from build123d import *


with BuildPart() as part:
    # Esquisse1 → Révolution1 (revolve)
    with BuildSketch(Plane.XY, mode=Mode.PRIVATE) as r_volution1_sk:
        Polygon((0, 45.2), (0, 50.8), (-0.2, 51), (-22.267949192, 51), (-24, 54), (-24, 67.8), (-24.2, 68), (-37.8, 68), (-38, 67.8), (-38, 58), (-47.8, 58), (-48, 57.8), (-48, 45.2), (-47.8, 45), (-0.2, 45), align=None)
    revolve(r_volution1_sk.sketch.rotate(Axis((0, 0, 0), (-1, 0, 0)), 90), axis=Axis((0, 0, 0), (-1, 0, 0)))  # turned: the seam where the file's is


solid = part.part
Model file for the job. Use its own axes, mm. A direction names the side the tool comes from. Give positions to 0.01 mm unless a question says otherwise; leave off trailing zeros. Write each loop counter-clockwise with the first axis right and the second up, starting at its lowest first coordinate (ties: lowest second). Pieces come first, ordered by that corner, then holes. Notation, with made-up numbers: (-23.75, -16) -> (-18.75, -16) arc R21 ccw to (-18.75, 17) -> close; hole circle Ø5 at (-35.5, 14). An arc over 180 degrees is marked (long way). Write item = value, one per line.
(1) Slice it at C-C, the plane x = -32. Give the cut face in (y, z), then the cut area to 4 significant figures.
Determined:
outline = circle Ø136 at (0, 0); hole circle Ø90 at (0, 0)
area = 8,165 mm2
(2) Mould opens along Y. For faces 4 (the face through (-22.376, 49.97, 11.096)), 5 (the face through (-38, -30, -50)), 6 (the face through (-23.667, 39.923, -20.765)) say: released by +Y, released by -Y, zero draft, split by the parting line, or undercut.
Determined:
face_4 = split by the parting line
face_5 = zero draft
face_6 = undercut
(3) Flat gauge pins, fed straight in: P1, Ø6, axis at x = -35.5, y = -49.5, coming from the -Z side; P2, Ø8, axis at x = -9.5, y = -47.5, coming from the -Z side; P3, Ø4, axis at x = -29, z = 42.5, coming from the -Y side. Where does each tip first touch, or does it go through?
Determined:
P1 = -49.62
P2 = -26.62
P3 = -54.62
(4) Probe line 1 along Y through (x, z) = (-10, 0); line 2 along Y through (x, z) = (-37, 0); line 3 along Z through (x, y) = (-21, 2). List the from-to ranges inside material, lowest first.
Determined:
line_1 = -51 to -45, 45 to 51
line_2 = -68 to -45, 45 to 68
line_3 = -50.96 to -44.96, 44.96 to 50.96
(5) Slice it at D-D, the plane x = -4. Give the cut face in (y, z).
Determined:
outline = circle Ø102 at (0, 0); hole circle Ø90 at (0, 0)
(6) Tool access for faces 1 (the face through (0, 29.9, -34.1)), 2 (the face through (-42.97, 51.46, -26.76)), 3 (the face through (-24, 30, -46)): list every direction of +Z, -Z, +X, -X, +Y, -Y with a clear straight run to the whole face (end or side of a thin tool).
Determined:
face_1 = +Z, -Z, +X, +Y, -Y
face_2 = -X
face_3 = +X
